```python
from build123d import *

# Parameters (mm, degrees)
SKETCH1_W           = 56
SKETCH1_H           = 64.5
BOSS_EXTRUDE1_DEPTH = 25.25
SKETCH2_W           = 51.4
SKETCH2_H           = 62.2
CUT_EXTRUDE1_DEPTH  = 50.614765947
FILLET1_R           = 1
FILLET3_R           = 12.75
SKETCH4_W           = 45.38697638
SKETCH4_H           = 20.5
CUT_EXTRUDE3_DEPTH  = 75.710999554
SKETCH5_R           = 4
SKETCH5_R_2         = 1.5
CUT_EXTRUDE4_DEPTH  = 70.380292591


with BuildPart() as part:
    # Sketch1 → Boss-Extrude1 (new body)
    with BuildSketch(Plane.XY):
        Rectangle(SKETCH1_W, SKETCH1_H)
    extrude(amount=BOSS_EXTRUDE1_DEPTH)

    # Sketch2 → Cut-Extrude1 (cut, through all)
    with BuildSketch(Plane.XY.offset(25.25)):
        with Locations((0, 1.15)):
            Rectangle(SKETCH2_W, SKETCH2_H)
    extrude(amount=-CUT_EXTRUDE1_DEPTH, mode=Mode.SUBTRACT)

    # Fillet1
    fillet1_edges = [part.edges().sort_by_distance(p)[0] for p in [
        (-25.7, -29.95, 12.625),
        (25.7, -29.95, 12.625),
        (28, -32.25, 12.625),
        (-28, -32.25, 12.625),
    ]]
    fillet(fillet1_edges, radius=FILLET1_R)

    # Fillet3
    # the kernel refuses this fillet: 12.75 mm, written as the material it takes off along each edge
    with BuildSketch(Plane(origin=(-59.875, 32.25, 25.25), x_dir=(0, 0, -1), z_dir=(1, 0, 0)), Plane(origin=(-6.175, 32.25, 25.25), x_dir=(0, 0, -1), z_dir=(1, 0, 0)), Plane(origin=(-59.875, 32.25, 0), x_dir=(0, -1, 0), z_dir=(1, 0, 0)), Plane(origin=(-6.175, 32.25, 0), x_dir=(0, -1, 0), z_dir=(1, 0, 0))) as fillet3_piece_1:
        with BuildLine():
            CenterArc((FILLET3_R, -FILLET3_R), FILLET3_R, 90, 90)
            Line((0, -FILLET3_R), (0, 0))
            Line((0, 0), (FILLET3_R, 0))
        make_face()
    extrude(amount=66.05, mode=Mode.SUBTRACT)

    # Sketch4 → Cut-Extrude3 (cut, through all)
    with BuildSketch(Plane.XZ.offset(32.25)):
        with Locations((0, 12.625)):
            Rectangle(SKETCH4_W, SKETCH4_H)
    extrude(amount=-CUT_EXTRUDE3_DEPTH, mode=Mode.SUBTRACT)

    # Sketch5 → Cut-Extrude4 (cut, through all)
    with BuildSketch(Plane.ZY.offset(28)):
        with Locations(Location((12.625, 19.54938724, 0), (0, 0, 270))):
            Circle(SKETCH5_R)
        with Locations(Location((12.625, 26.54938724, 0), (0, 0, 270))):
            Circle(SKETCH5_R_2)
        with Locations(Location((19.625, 19.54938724, 0), (0, 0, 270))):
            Circle(SKETCH5_R_2)
        with Locations(Location((12.625, 12.54938724, 0), (0, 0, 270))):
            Circle(SKETCH5_R_2)
        with Locations(Location((5.625, 19.54938724, 0), (0, 0, 270))):
            Circle(SKETCH5_R_2)
    extrude(amount=-CUT_EXTRUDE4_DEPTH, mode=Mode.SUBTRACT)


solid = part.part
```
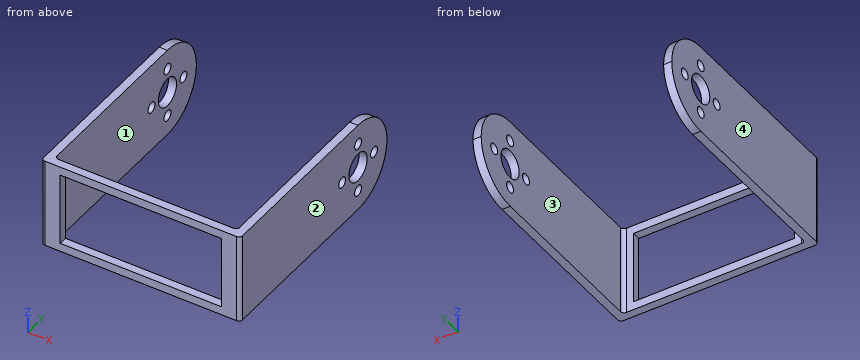
Read the model definition and answer for the solid it produces. Units are mm, in the model's axes. Face numbers are marked on the shaded views. Give positions to 0.01 mm unless a question says otherwise; leave off trailing zeros. Order: outer loops, then holes, each group sorted by start corner. A loop starts at its lowest first (then second) coordinate and runs counter-clockwise, first axis right, second up. Notation, with made-up numbers: (87.5, -13) -> (103.5, -13) arc R30 ccw to (103.5, 16) -> close; hole circle Ø2 at (49.5, 26). An arc over 180 degrees is marked (long way). Write item = value, one per line.
1. A cutting plane is placed at B-B, the plane x = 8. Write down the section's boundary in (y, z) (3 decimals), and give its area (3 significant figures).
Numbers:
outline = (-32.25, 0) -> (-29.95, 0) -> (-29.95, 2.375) -> (-32.25, 2.375) -> close; (-32.25, 22.875) -> (-29.95, 22.875) -> (-29.95, 25.25) -> (-32.25, 25.25) -> close
area = 10.9 mm²
2. A cutting plane is placed at A-A, the plane y = -11. Write down the section's boundary in (x, z), and give its area (3 significant figures).
Numbers:
outline = (-28, 0) -> (-25.7, 0) -> (-25.7, 25.25) -> (-28, 25.25) -> close; (25.7, 0) -> (28, 0) -> (28, 25.25) -> (25.7, 25.25) -> close
area = 116 mm²
3. The mould has two halves that part along X. Classify the marked faces 1, 2, 3 and 4: +X half, -X half, draft (parallel to the pull), parting line (faces both ways), or undercut.
Numbers:
face_1 = undercut
face_2 = +X half
face_3 = undercut
face_4 = -X half
4. A cutting plane is placed at C-C, the plane y = 26. Write down the section's boundary in (x, z), and give its area (3 significant figures).
Numbers:
outline = (-28, 1.78) -> (-25.7, 1.78) -> (-25.7, 11.23) -> (-28, 11.23) -> close; (-28, 14.02) -> (-25.7, 14.02) -> (-25.7, 23.47) -> (-28, 23.47) -> close; (25.7, 1.78) -> (28, 1.78) -> (28, 11.23) -> (25.7, 11.23) -> close; (25.7, 14.02) -> (28, 14.02) -> (28, 23.47) -> (25.7, 23.47) -> close
area = 86.9 mm²
5. A cutting plane is placed at D-D, the plane y = 17. Write down the section's boundary in (x, z), and give its area (3 significant figures).
Numbers:
outline = (-28, 0) -> (-25.7, 0) -> (-25.7, 9.54) -> (-28, 9.54) -> close; (-28, 15.71) -> (-25.7, 15.71) -> (-25.7, 25.25) -> (-28, 25.25) -> close; (25.7, 0) -> (28, 0) -> (28, 9.54) -> (25.7, 9.54) -> close; (25.7, 15.71) -> (28, 15.71) -> (28, 25.25) -> (25.7, 25.25) -> close
area = 87.8 mm²
6. Given pin 1 (5 mm diameter, centred on x = 0, z = 20.5, fed in from +Y), flat-ended and moving along its own axis, determine where the tip first touches the part or whether it passes through.
Numbers:
pin_1 = -29.95
7. Straight lines are drawn through the part: line 1 along X through (y, z) = (-24, 21.25); line 2 along Y through (x, z) = (-10, 23.25); line 3 along Y through (x, z) = (25, 2). For each, find the intervals that lie inside material, in ascending order.
Numbers:
line_1 = -28 to -25.7, 25.7 to 28
line_2 = -32.25 to -29.95
line_3 = -32.25 to -29.9
